from build123d import *

# Parameters (mm, degrees)
F2_R     = 38.1
F3_DEPTH = 82.55
F3_TAPER = 6
F4_SIZE  = 3.81
F5_R     = 1.27
F6_R     = 1.27


with BuildPart() as f1:
    # F0 (on Front) → F1 (revolve)
    with BuildSketch(Plane.XZ):
        Polygon((-60.6646513261, 41.275), (-60.6646513261, 0), (40.9353486739, 0), (40.9353486739, 34.7477929017), (32.8286082969, 35.2272205055), (29.094543308, 31.804330647), (25.956897065, 35.2272205055), (12.8358363484, 35.2272205055), (8.2719782367, 31.804330647), (5.7048136368, 35.2272205055), align=None)
    revolve(axis=Axis((-9.8646513261, 0, 0), (-1, 0, 0)))

    # F2 (on face) → F3 (cut)
    with BuildSketch(Plane(origin=(-60.6646513261, 0, 0), x_dir=(0, -1, 0), z_dir=(-1, 0, 0))):
        Circle(F2_R)
    extrude(amount=-F3_DEPTH, taper=F3_TAPER, mode=Mode.SUBTRACT)

    # F4
    f4_edges = [f1.edges().sort_by_distance(p)[0] for p in [
        (40.935349, 0, -34.747793),
    ]]
    chamfer(f4_edges, length=F4_SIZE)

    # F5
    f5_edges = [f1.edges().sort_by_distance(p)[0] for p in [
        (-60.664651, 0, -41.275),
    ]]
    fillet(f5_edges, radius=F5_R)

    # F6
    f6_edges = [f1.edges().sort_by_distance(p)[0] for p in [
        (-60.664651, 0, -39.884012),
        (-60.664651, 38.1, 0),
    ]]
    fillet(f6_edges, radius=F6_R)


solid = f1.part
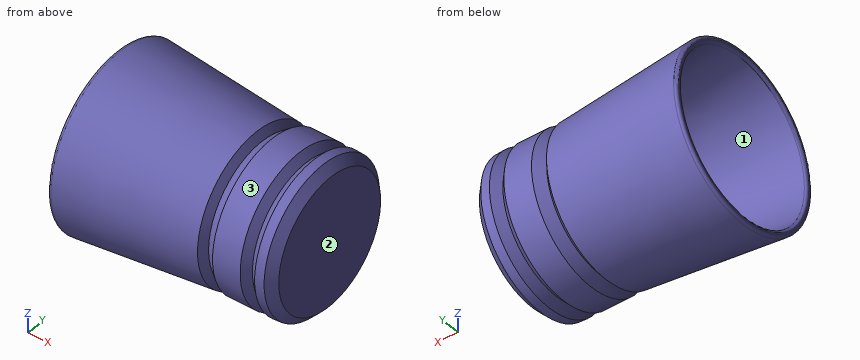
Read the model definition and answer for the solid it produces. Units are mm, in the model's axes. Face numbers are marked on the shaded views. Coordinates: 2 decimals unless noted, no trailing zeros. Order: outer loops, then holes, each group sorted by start corner. A loop starts at its lowest first (then second) coordinate and runs counter-clockwise, first axis right, second up. Notation, with made-up numbers: (57.25, 75.5) -> (66.25, 75.5) arc R36 cw to (66.25, 113.5) -> close; hole circle Ø2 at (-15, 42). An arc over 180 degrees is marked (long way). Answer as a JSON object with one key per item and string values.
1) A cutting plane is placed at A-A, the plane y = 0. Determine the outline of the cut face in (x, z), plus the area to 3 significant figures.
Model answer:
{"outline": "(-60.66, -39.88) arc R1.27 ccw to (-59.28, -41.15) -> (5.7, -35.23) -> (8.27, -31.8) -> (12.84, -35.23) -> (25.96, -35.23) -> (29.09, -31.8) -> (32.83, -35.23) -> (37.13, -34.97) -> (40.94, -30.94) -> (40.94, 30.94) -> (37.13, 34.97) -> (32.83, 35.23) -> (29.09, 31.8) -> (25.96, 35.23) -> (12.84, 35.23) -> (8.27, 31.8) -> (5.7, 35.23) -> (-59.28, 41.15) arc R1.27 ccw to (-60.66, 39.88) -> (-60.66, 39.24) arc R1.27 ccw to (-59.53, 37.98) -> (21.89, 29.42) -> (21.89, -29.42) -> (-59.53, -37.98) arc R1.27 ccw to (-60.66, -39.24) -> close", "area": "1,920 mm²"}
2) Each of these flat-tipped pins is pushed along its axis until it touches: pin 1 (1.5 mm diameter, centred on x = -36, y = -4, fed in from -Z); pin 2 (6 mm diameter, centred on y = 24.5, z = 3, fed in from -X); pin 3 (10 mm diameter, centred on y = 18.5, z = 29, fed in from +X); pin 4 (3 mm diameter, centred on x = 0.5, z = -19.5, fed in from -Y). Where does it stop, or does it pass through?
Model answer:
{"pin 1": "stops at z = -38.92", "pin 2": "stops at x = 21.89", "pin 3": "stops at x = 40.94", "pin 4": "stops at y = -30.85"}
3) Consider line 1 along X through (y, z) = (18, -10.5); line 2 along Z through (x, y) = (-46, 8); line 3 along Y through (x, z) = (-51, 20). Determine where each line is inside the solid, lowest interval first. Write a range as from..to.
Model answer:
{"line 1": "x = 21.89..40.94", "line 2": "z = -39.13..-35.67, 35.67..39.13", "line 3": "y = -35.1..-31.23, 31.23..35.1"}
4) The mould has two halves that part along Z. Classify the marked faces 1, 2 and 3: released by +Z, released by -Z, zero draft, split by the parting line, or undercut.
Model answer:
{"face 1": "undercut", "face 2": "zero draft", "face 3": "split by the parting line"}
5) A cutting plane is placed at B-B, the plane x = -38.5. Determine the outline of the cut face in (y, z), plus the area to 3 significant figures.
Model answer:
{"outline": "circle Ø78.51 at (0, 0); hole circle Ø71.54 at (0, 0)", "area": "821 mm²"}
